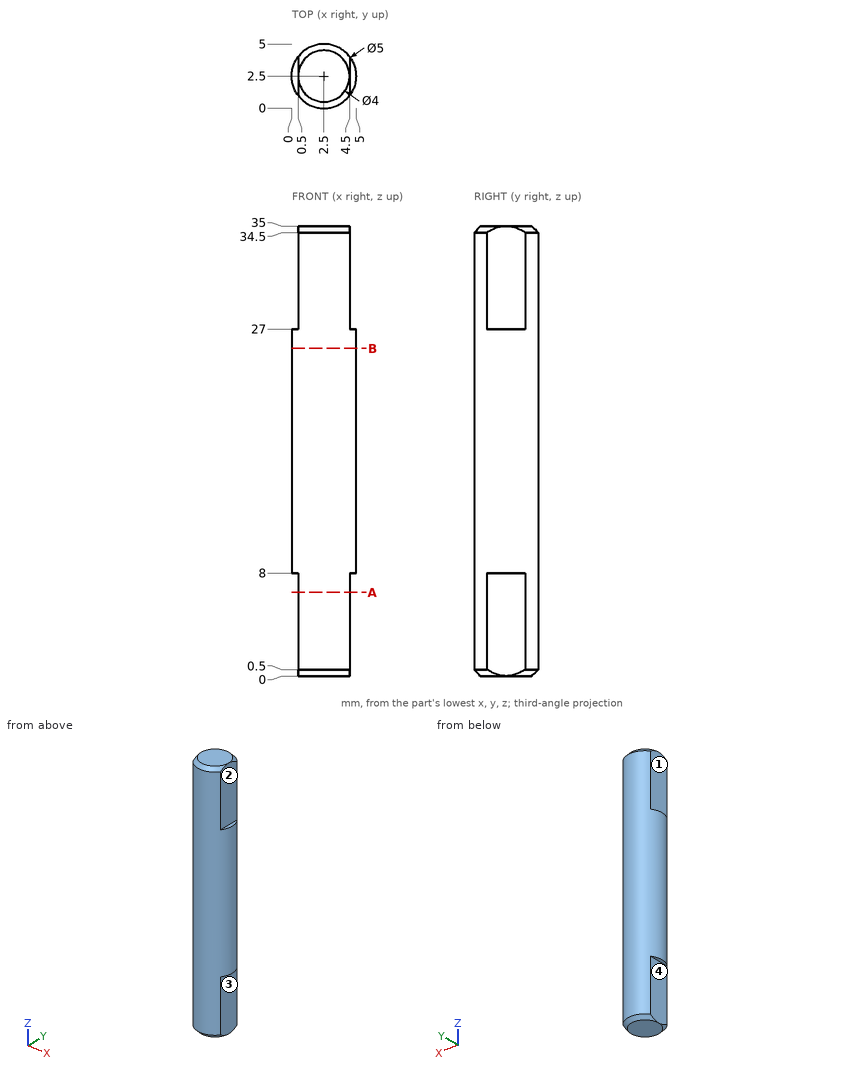
Answer from the drawing. Dimensions are ordinates in mm from the lowest x, y and z of the part. A direction names the side the tool comes from. Coordinates: 2 decimals unless noted, no trailing zeros. Write each loop counter-clockwise with the first axis right and the second up, starting at its lowest first coordinate (ties: lowest second). Pieces come first, ordered by that corner, then holes. Notation, with made-up numbers: M -1.75,18.5 L 2.25,18.5 A5 ccw 2.25,24.5 Z; hole C 84.25,47 d1. An arc over 180 degrees is marked long. Use a Markdown table: item, result.
Q1. The part is cut by section B-B, the plane z = 25.5. Write down the section's boundary in (x, y).
Answer block:
| item | result |
|---|---|
| outline | C 2.5,2.5 d5 |
Q2. The part is cut by section A-A, the plane z = 6.5. Write down the section's boundary in (x, y).
Answer block:
| item | result |
|---|---|
| outline | M 0.5,1 A2.5 ccw 4.5,1 L 4.5,4 A2.5 ccw 0.5,4 Z |
Q3. Each of these flat-tipped pins is pushed along its axis until it touches: pin 1 Ø0.6 at (x, y) = (0, 2.5) entering from -Z; pin 2 Ø2.5 at (y, z) = (3, 32) entering from +X; pin 3 Ø3 at (x, z) = (1, 8) entering from +Y; pin 4 Ø2.5 at (y, z) = (2, 3.5) entering from -X. Where does it stop, or does it pass through?
Answer block:
| item | result |
|---|---|
| pin 1 | stops at z = 8 |
| pin 2 | stops at x = 4.5 |
| pin 3 | stops at y = 5 |
| pin 4 | stops at x = 0.5 |
Q4. Straight lines are drawn through the part: L1, parallel to X at y = 3.9, z = 30.5; L2, parallel to Y at x = 3.15, z = 18; L3, parallel to X at y = 3, z = 25. For each, find the intervals that lie inside material, in ascending order. Write a range as [from, to].
Answer block:
| item | result |
|---|---|
| L1 | x = [0.5, 4.5] |
| L2 | y = [0.09, 4.91] |
| L3 | x = [0.05, 4.95] |
Q5. Which of the six approach directions +Z, -Z, +X, -X, +Y, -Y give full straight-line access (tool end or side, diameter ignored) to the marked faces 1, 2, 3 and 4?
Answer block:
| item | result |
|---|---|
| face 1 | +Z, -X, +Y, -Y |
| face 2 | +Z, +X, +Y, -Y |
| face 3 | -Z, +X, +Y, -Y |
| face 4 | -Z, -X, +Y, -Y |
